Check sheet for the modelled part. Datum: model origin and axes. Units: mm. A direction names the side the tool comes from. Give positions to 0.01 mm unless a question says otherwise; leave off trailing zeros. Write each loop counter-clockwise with the first axis right and the second up, starting at its lowest first coordinate (ties: lowest second). Pieces come first, ordered by that corner, then holes. Notation, with made-up numbers: (63, 61.5) -> (119, 61.5) arc R11 ccw to (119, 65.5) -> close; hole circle Ø10 at (-3.75, 29). An arc over 180 degrees is marked (long way). Return JSON: item names as keys, results as strings.
from build123d import *

# Parameters (mm, degrees)
F0_R     = 7
F0_R_2   = 5.5
F1_DEPTH = 23.5
F2_DEPTH = 23.45
F3_R     = 4.5
F4_DEPTH = 0.3
F5_R     = 2.5
F6_DEPTH = 2


with BuildPart() as f1:
    # F0 (on Front) → F1 (new body, symmetric)
    with BuildSketch(Plane.XZ):
        Circle(F0_R)
        Circle(F0_R_2, mode=Mode.SUBTRACT)
    extrude(amount=F1_DEPTH, both=True)

    # F0 (on Front) → F2 (join, symmetric)
    with BuildSketch(Plane.XZ):
        Circle(F0_R_2)
    extrude(amount=F2_DEPTH, both=True)

    # F3 (on face) → F4 (join)
    with BuildSketch(Plane.XZ.offset(23.45)):
        Circle(F3_R)
    extrude(amount=F4_DEPTH)

    # F5 (on face) → F6 (join)
    with BuildSketch(Plane(origin=(0, 23.45, 0), x_dir=(-1, 0, 0), z_dir=(0, 1, 0))):
        Circle(F5_R)
    extrude(amount=F6_DEPTH)


solid = f1.part
(1) Cross-section at A-A on z = 0. Enter the section's corners in (x, y), then the cut area to 3 significant figures.
Reply:
{"outline": "(-7, -23.5) -> (-5.5, -23.5) -> (-5.5, -23.45) -> (-4.5, -23.45) -> (-4.5, -23.75) -> (4.5, -23.75) -> (4.5, -23.45) -> (5.5, -23.45) -> (5.5, -23.5) -> (7, -23.5) -> (7, 23.5) -> (5.5, 23.5) -> (5.5, 23.45) -> (2.5, 23.45) -> (2.5, 25.45) -> (-2.5, 25.45) -> (-2.5, 23.45) -> (-5.5, 23.45) -> (-5.5, 23.5) -> (-7, 23.5) -> close", "area": "670 mm^2"}
(2) Cross-section at C-C on y = -9. Enter the section's corners in (x, z), then the cut area to 3 significant figures.
Reply:
{"outline": "circle Ø14 at (0, 0)", "area": "154 mm^2"}
(3) Depth check by flat-ended pin: pin 1 Ø1 at (x, y) = (-4, 18) entering from +Z; pin 2 Ø3 at (x, y) = (-4, 8.5) entering from +Z; pin 3 Ø1.5 at (x, z) = (4, 4.5) entering from +Y. Enter the tip coordinate at first touch or a pass-through.
Reply:
{"pin 1": "z = 6.06", "pin 2": "z = 6.54", "pin 3": "y = 23.5"}
(4) Cross-section at D-D on x = -3.5. Enter the section's corners in (y, z), then the cut area to 3 significant figures.
Reply:
{"outline": "(-23.75, -2.83) -> (-23.45, -2.83) -> (-23.45, -4.24) -> (-23.5, -4.24) -> (-23.5, -6.06) -> (23.5, -6.06) -> (23.5, -4.24) -> (23.45, -4.24) -> (23.45, 4.24) -> (23.5, 4.24) -> (23.5, 6.06) -> (-23.5, 6.06) -> (-23.5, 4.24) -> (-23.45, 4.24) -> (-23.45, 2.83) -> (-23.75, 2.83) -> close", "area": "571 mm^2"}
(5) Release check for a two-part mould opening along Z. For faces 4 (the cylindrical face through (-3.32, -23.6, 3.04)), 5 (the cylindrical face through (6.466, -0.329, -2.681)), 6 (the flat face through (0, 25.45, 0)) record: pulls with the +Z half, pulls with the -Z half, needs draft (parallel to the pull), parting line crosses it, or undercut.
Reply:
{"face 4": "undercut", "face 5": "parting line crosses it", "face 6": "needs draft"}
(6) Thickness scan on L1, parallel to Z at x = 0, y = 23.55; L2, parallel to X at y = 0.5, z = 0.25; L3, parallel to Y at x = -4.25, z = 3.75. Record the ranges inside material, lowest first.
Reply:
{"L1": "-2.5 to 2.5", "L2": "-7 to 7", "L3": "-23.5 to 23.5"}
(7) Cross-section at B-B on x = 0. Enter the section's corners in (y, z).
Reply:
{"outline": "(-23.75, -4.5) -> (-23.45, -4.5) -> (-23.45, -5.5) -> (-23.5, -5.5) -> (-23.5, -7) -> (23.5, -7) -> (23.5, -5.5) -> (23.45, -5.5) -> (23.45, -2.5) -> (25.45, -2.5) -> (25.45, 2.5) -> (23.45, 2.5) -> (23.45, 5.5) -> (23.5, 5.5) -> (23.5, 7) -> (-23.5, 7) -> (-23.5, 5.5) -> (-23.45, 5.5) -> (-23.45, 4.5) -> (-23.75, 4.5) -> close"}
(8) Set-up check for faces 1 (the flat face through (0, -23.75, 0)), 2 (the flat face through (-5, -23.45, 0)), 3 (the cylindrical face through (0.54, 24.44, -2.44)): record each of +Z, -Z, +X, -X, +Y, -Y from which the full face is reachable in a straight line by a thin tool's end or side.
Reply:
{"face 1": "+Z, -Z, +X, -X, -Y", "face 2": "-Y", "face 3": "+Y"}
